```python
from build123d import *

# Parameters (mm, degrees)
BOSS_EXTRUDE2_DEPTH = 10
SKETCH4_R           = 4
CUT_EXTRUDE1_DEPTH  = 4
FILLET1_R           = 3
SKETCH5_R           = 1.75
SKETCH5_R_2         = 3.31
CUT_EXTRUDE2_DEPTH  = 10
SKETCH7_R           = 1.75
CUT_EXTRUDE3_DEPTH  = 10
SKETCH8_R           = 3.5
CUT_EXTRUDE4_DEPTH  = 3


with BuildPart() as part:
    # Sketch1 → Boss-Extrude2 (new body)
    with BuildSketch(Plane(origin=(0, 0, 0), x_dir=(1, 0, 0), z_dir=(0, 1, 0))):
        Polygon((0, 0), (10, -45), (50, -45), (60, 0), align=None)
    extrude(amount=BOSS_EXTRUDE2_DEPTH)

    # Sketch4 → Cut-Extrude1 (cut)
    with BuildSketch(Plane(origin=(0, 10, 0), x_dir=(1, 0, 0), z_dir=(0, 1, 0))):
        with Locations(Location((15, -6.5, 0), (0, 0, 270))):
            Circle(SKETCH4_R)
        with Locations(Location((45, -6.5, 0), (0, 0, 270))):
            Circle(SKETCH4_R)
        with Locations(Location((45, -36.5, 0), (0, 0, 270))):
            Circle(SKETCH4_R)
        with Locations(Location((15, -36.5, 0), (0, 0, 270))):
            Circle(SKETCH4_R)
    extrude(amount=-CUT_EXTRUDE1_DEPTH, mode=Mode.SUBTRACT)

    # Fillet1
    fillet1_edges = [part.edges().sort_by_distance(p)[0] for p in [
        (60, 5, 0),
        (50, 5, 45),
        (10, 5, 45),
        (0, 5, 0),
    ]]
    fillet(fillet1_edges, radius=FILLET1_R)

    # Sketch5 → Cut-Extrude2 (cut)
    with BuildSketch(Plane.XZ):
        with Locations(Location((12, 21, 0), (0, 0, 270))):
            Circle(SKETCH5_R)
        with Locations(Location((48, 21, 0), (0, 0, 270))):
            Circle(SKETCH5_R)
        with Locations(Location((30, 21, 0), (0, 0, 270))):
            Circle(SKETCH5_R_2)
    extrude(amount=-CUT_EXTRUDE2_DEPTH, mode=Mode.SUBTRACT)

    # Sketch7 → Cut-Extrude3 (cut)
    with BuildSketch(Plane(origin=(0, 10, 0), x_dir=(1, 0, 0), z_dir=(0, 1, 0))):
        with Locations(Location((15, -6.5, 0), (0, 0, 270))):
            Circle(SKETCH7_R)
        with Locations(Location((45, -6.5, 0), (0, 0, 270))):
            Circle(SKETCH7_R)
        with Locations(Location((45, -36.5, 0), (0, 0, 270))):
            Circle(SKETCH7_R)
        with Locations(Location((15, -36.5, 0), (0, 0, 270))):
            Circle(SKETCH7_R)
    extrude(amount=-CUT_EXTRUDE3_DEPTH, mode=Mode.SUBTRACT)

    # Sketch8 → Cut-Extrude4 (cut)
    with BuildSketch(Plane.XZ):
        with Locations(Location((15, 36.5, 0), (0, 0, 270))):
            Circle(SKETCH8_R)
        with Locations(Location((45, 36.5, 0), (0, 0, 270))):
            Circle(SKETCH8_R)
        with Locations(Location((45, 6.5, 0), (0, 0, 270))):
            Circle(SKETCH8_R)
        with Locations(Location((15, 6.5, 0), (0, 0, 270))):
            Circle(SKETCH8_R)
    extrude(amount=-CUT_EXTRUDE4_DEPTH, mode=Mode.SUBTRACT)


solid = part.part
```
Geometry: final body of the model. Coordinates: model frame, mm. A direction names the side the tool comes from. Round coordinates to 2 decimals unless told otherwise and drop trailing zeros. Order: outer loops, then holes, each group sorted by start corner. A loop starts at its lowest first (then second) coordinate and runs counter-clockwise, first axis right, second up. Notation, with made-up numbers: M 63,23.25 L 72,23.25 A34 ccw 72,58.25 Z; hole C 40,47.25 d5. An arc over 180 degrees is marked long. Use one line per item in the form item = value. Start each with the question number.
Q1. Cut plane A-A (x = 45). Return loops of the section in (y, z).
Q2. Pin query (flat end, axial travel): pin 1 Ø5 at (y, z) = (8.5, 38) entering from +X; pin 2 Ø2 at (x, z) = (16, 36) entering from -Y; pin 3 Ø2 at (y, z) = (5, 26.5) entering from +X; pin 4 Ø2 at (x, z) = (48, 21) entering from -Y. Return the tip coordinate at first contact, or that it passes through.
Q3. Cut plane B-B (y = 9.25). Return loops of the section in (x, z).
Q4. Material intervals for line 1 (X direction, y = 5, z = 36.5); line 2 (X direction, y = 1.45, z = 36.5); line 3 (X direction, y = 5.25, z = 21), sorted ascending. Write a range as [from, to].
Q5. Access query for faces 4 (the face through (17, 3, 36)), 5 (the face through (14.17, 6, 38.22)), 6 (the face through (49.448, 5.07, 44.358)). Directions: +Z, -Z, +X, -X, +Y, -Y. A direction counts if a zero-diameter tool reaches every point of the face in a straight line with its end or side. Return the directions, or none.
Q6. Cut plane C-C (x = 30). Return loops of the section in (y, z), and give its area (3 significant figures).
Q7. Mould query, pull axis X, two halves, no side actions, for faces 1 (the face through (10.507, 5.07, 44.322)), 2 (the face through (47, 3, 6)), 3 (the face through (54.8, 4.9, 23.4)). Classes: +X half, -X half, draft (parallel to the pull), parting line (faces both ways), or undercut.
Q8. Cut plane D-D (z = 21). Return loops of the section in (x, y).
Geometry results:
q1.outline = M 0,0 L 10,0 L 10,2.5 L 6,2.5 L 6,4.75 L 3,4.75 L 3,3 L 0,3 Z; M 0,10 L 3,10 L 3,8.25 L 6,8.25 L 6,10.5 L 10,10.5 L 10,32.5 L 6,32.5 L 6,34.75 L 3,34.75 L 3,33 L 0,33 Z; M 0,40 L 3,40 L 3,38.25 L 6,38.25 L 6,40.5 L 10,40.5 L 10,45 L 0,45 Z
q2.pin_1 = 52.11
q2.pin_2 = 3
q2.pin_3 = 54.33
q2.pin_4 = through
q3.outline = M 0.81,3.65 A3 ccw 3.74,0 L 56.26,0 A3 ccw 59.19,3.65 L 50.52,42.65 A3 ccw 47.59,45 L 12.41,45 A3 ccw 9.48,42.65 Z; hole C 12,21 d3.5; hole C 15,6.5 d8; hole C 15,36.5 d8; hole C 30,21 d6.62; hole C 45,6.5 d8; hole C 45,36.5 d8; hole C 48,21 d3.5
q4.line_1 = [8.11, 13.25], [16.75, 43.25], [46.75, 51.89]
q4.line_2 = [8.11, 11.5], [18.5, 41.5], [48.5, 51.89]
q4.line_3 = [4.67, 10.25], [13.75, 26.69], [33.31, 46.25], [49.75, 55.33]
q5.face_4 = -Y
q5.face_5 = +Y
q5.face_6 = +Z, +X, +Y, -Y
q6.outline = M 0,0 L 10,0 L 10,17.69 L 0,17.69 Z; M 0,24.31 L 10,24.31 L 10,45 L 0,45 Z
q6.area = 384 mm^2
q7.face_1 = -X half
q7.face_2 = undercut
q7.face_3 = +X half
q8.outline = M 4.67,0 L 10.25,0 L 10.25,10 L 4.67,10 Z; M 13.75,0 L 26.69,0 L 26.69,10 L 13.75,10 Z; M 33.31,0 L 46.25,0 L 46.25,10 L 33.31,10 Z; M 49.75,0 L 55.33,0 L 55.33,10 L 49.75,10 Z
